CAD build for the part. Positions are in the model's coordinates, mm. Face numbers are marked on the shaded views. A direction names the side the tool comes from. Round coordinates to 2 decimals unless told otherwise and drop trailing zeros. Write each loop counter-clockwise with the first axis right and the second up, starting at its lowest first coordinate (ties: lowest second). Pieces come first, ordered by that corner, then holes. Notation, with made-up numbers: (18.5, 86) - (40.5, 86) arc R18 cw to (40.5, 114) - close; hole circle Ø10 at (37.5, 77). An arc over 180 degrees is marked (long way). Answer in a Markdown table with one row per item.
```python
from build123d import *

# Parameters (mm, degrees)
PAD_DEPTH       = 26
POCKET_DEPTH    = 24
SKETCH002_R     = 8.25
POCKET001_DEPTH = 3
SKETCH003_R     = 5.5
POCKET002_DEPTH = 3
SKETCH004_R     = 1.75
POCKET003_DEPTH = 5


with BuildPart() as part:
    # Sketch → Pad (new body)
    with BuildSketch(Plane.XY):
        with BuildLine():
            Line((60, 8), (60, 82.000001))
            ThreePointArc((60, 82.000001), (58.434586, 89.869877), (53.976662, 96.541638))
            Line((40.541631, 109.976664), (53.976662, 96.541638))
            ThreePointArc((40.541631, 109.976664), (33.869872, 114.434584), (25.999999, 115.999997))
            Line((7.999999, 115.999997), (25.999999, 115.999997))
            ThreePointArc((7.999999, 115.999997), (2.343146, 113.656851), (0, 107.999998))
            Line((0, 107.999998), (0, 8))
            ThreePointArc((0, 8), (2.343146, 2.343146), (8, 0))
            Line((8, 0), (52, 0))
            ThreePointArc((52, 0), (57.656854, 2.343146), (60, 8))
        make_face()
    extrude(amount=PAD_DEPTH)

    # Sketch001 → Pocket (cut)
    with BuildSketch(Plane.XY.offset(26)):
        with BuildLine():
            ThreePointArc((8.00001, 113.999998), (3.757363, 112.242642), (2, 107.999998))
            Line((2, 107.999998), (2, 8))
            ThreePointArc((2, 8), (3.757359, 3.757359), (8, 2))
            Line((8, 2), (52, 2))
            ThreePointArc((52, 2), (56.242642, 3.757359), (58.000001, 8))
            Line((58.000001, 82), (58.000001, 8))
            ThreePointArc((58.000001, 82), (56.586824, 89.104519), (52.562435, 95.127438))
            Line((39.127419, 108.562437), (52.562435, 95.127438))
            ThreePointArc((39.127419, 108.562437), (33.104503, 112.586822), (25.99999, 113.999998))
            Line((8.00001, 113.999998), (25.99999, 113.999998))
        make_face()
    extrude(amount=-POCKET_DEPTH, mode=Mode.SUBTRACT)

    # Sketch002 → Pocket001 (cut)
    with BuildSketch(Plane(origin=(75.259141, 75.259166, 0), x_dir=(-0.707107, 0.707107, 0), z_dir=(0.707107, 0.707107, 0))):
        with Locations((39.5, 13)):
            Circle(SKETCH002_R)
    extrude(amount=-POCKET001_DEPTH, mode=Mode.SUBTRACT)

    # Sketch003 → Pocket002 (cut)
    with BuildSketch(Plane(origin=(0, 115.999997, 0), x_dir=(-1, 0, 0), z_dir=(0, 1, 0))):
        with Locations((-17, 13)):
            Circle(SKETCH003_R)
    extrude(amount=-POCKET002_DEPTH, mode=Mode.SUBTRACT)

    # Sketch004 → Pocket003 (cut)
    with BuildSketch(Plane.XY.offset(2)):
        with Locations((30, 29)):
            Circle(SKETCH004_R)
        with Locations((30, 57)):
            Circle(SKETCH004_R)
    extrude(amount=-POCKET003_DEPTH, mode=Mode.SUBTRACT)


solid = part.part
```
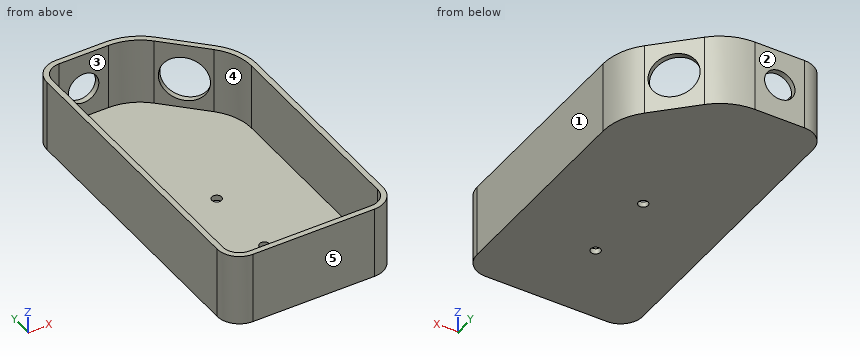
Q1. Flat gauge pins, fed straight in: pin 1 (12 mm diameter, centred on x = 17, y = 44.5, fed in from +Z); pin 2 (8 mm diameter, centred on x = 41.5, z = 15, fed in from +Y); pin 3 (10 mm diameter, centred on x = 17, z = 13, fed in from +Y). Where does each tip first touch, or does it go through?
Computed:
| item | result |
|---|---|
| pin 1 | stops at z = 2 |
| pin 2 | stops at y = 112.48 |
| pin 3 | stops at y = 2 |
Q2. 3-axis set-ups, long thin cutter, end or side, ignore diameter. For the marked faces 4 and 5: which of +Z, -Z, +X, -X, +Y, -Y reach the whole face in a straight line?
Computed:
| item | result |
|---|---|
| face 4 | +Z |
| face 5 | +Z, -Z, +X, -X, -Y |
Q3. Drill centre lines: line 1 (X direction, y = 8.5, z = 9.5); line 2 (Y direction, x = 30, z = 1.05); line 3 (Y direction, x = 11, z = 17). Where is each one in solid material? Low to high.
Computed:
| item | result |
|---|---|
| line 1 | x = 0 to 2, 58 to 60 |
| line 2 | y = 0 to 27.25, 30.75 to 55.25, 58.75 to 115.61 |
| line 3 | y = 0 to 2, 114 to 116 |
Q4. Saw through at A-A on y = 29. List the corners of the cut face in (x, z).
Computed:
| item | result |
|---|---|
| outline | (0, 0) - (28.25, 0) - (28.25, 2) - (2, 2) - (2, 26) - (0, 26) - close; (31.75, 0) - (60, 0) - (60, 26) - (58, 26) - (58, 2) - (31.75, 2) - close |
Q5. Saw through at B-B on z = 13. List the corners of the cut face in (x, y) (1 decimal).
Computed:
| item | result |
|---|---|
| outline | (0, 8) arc R8 ccw to (8, 0) - (52, 0) arc R8 ccw to (60, 8) - (60, 82) arc R20.6 ccw to (54, 96.5) - (53.2, 97.4) - (51.7, 95.9) - (52.6, 95.1) arc R18.6 cw to (58, 82) - (58, 8) arc R6 cw to (52, 2) - (8, 2) arc R6 cw to (2, 8) - (2, 108) arc R6 cw to (8, 114) - (11.5, 114) - (11.5, 116) - (8, 116) arc R8 ccw to (0, 108) - close; (22.5, 114) - (26, 114) arc R18.6 cw to (39.1, 108.6) - (40.1, 107.6) - (41.5, 109) - (40.5, 110) arc R20.6 ccw to (26, 116) - (22.5, 116) - close |
Q6. Saw through at C-C on x = 17.5. List the corners of the cut face in (y, z), then the cut area to 3 significant figures.
Computed:
| item | result |
|---|---|
| outline | (0, 0) - (116, 0) - (116, 7.52) - (114, 7.52) - (114, 2) - (2, 2) - (2, 26) - (0, 26) - close; (114, 18.48) - (116, 18.48) - (116, 26) - (114, 26) - close |
| area | 306 mm2 |
Q7. Saw through at D-D on y = 47.5. List the corners of the cut face in (x, z), then the cut area to 3 significant figures.
Computed:
| item | result |
|---|---|
| outline | (0, 0) - (60, 0) - (60, 26) - (58, 26) - (58, 2) - (2, 2) - (2, 26) - (0, 26) - close |
| area | 216 mm2 |
Q8. Pull direction Y, two halves, no side cores. Call the marked faces 1, 2 and 3: released by +Y, released by -Y, zero draft, split by the parting line, or undercut.
Computed:
| item | result |
|---|---|
| face 1 | zero draft |
| face 2 | released by +Y |
| face 3 | undercut |
